Work out the finished part from the listing and answer in its coordinate system (mm). A direction names the side the tool comes from. Give positions to 0.01 mm unless a question says otherwise; leave off trailing zeros. Loops run counter-clockwise (first coordinate to the right, second up) from the corner with the lowest first, then second, coordinate; pieces in that order, holes last. Notation, with made-up numbers: (-30, 5.25) - (3, 5.25) arc R17 cw to (3, 30.25) - close; hole circle Ø7 at (-37.5, 17.25). An arc over 180 degrees is marked (long way). One line per question, with ' | ' between items.
from build123d import *

# Parameters (mm, degrees)
CROQUIS1_R              = 10
SALIENTE_EXTRUIR1_DEPTH = 75
CROQUIS2_R              = 11
SALIENTE_EXTRUIR2_DEPTH = 2
CROQUIS3_W              = 15
CROQUIS3_H              = 10
SALIENTE_EXTRUIR3_DEPTH = 5


with BuildPart() as part:
    # Croquis1 → Saliente-Extruir1 (new body)
    with BuildSketch(Plane.XY):
        Circle(CROQUIS1_R)
    extrude(amount=SALIENTE_EXTRUIR1_DEPTH)

    # Croquis2 → Saliente-Extruir2 (add)
    with BuildSketch(Plane.XY.offset(75)):
        Circle(CROQUIS2_R)
    extrude(amount=SALIENTE_EXTRUIR2_DEPTH)

    # Croquis3 → Saliente-Extruir3 (add)
    with BuildSketch(Plane(origin=(0, 0, 0), x_dir=(-1, 0, 0), z_dir=(0, 0, -1))):
        Rectangle(CROQUIS3_W, CROQUIS3_H)
    extrude(amount=SALIENTE_EXTRUIR3_DEPTH)


solid = part.part
1. Find section C-C on z = 19. Write down the section's boundary in (x, y), then the cut area to 3 significant figures.
Evaluation:
outline: circle Ø20 at (0, 0) | area: 314 mm2
2. Find section D-D on y = 7.25. Write down the section's boundary in (x, z), then the cut area to 3 significant figures.
Evaluation:
outline: (-8.27, 75) - (-6.89, 75) - (-6.89, 0) - (6.89, 0) - (6.89, 75) - (8.27, 75) - (8.27, 77) - (-8.27, 77) - close | area: 1,070 mm2
3. Flat-ended cylindrical pins translate along their axes: pin 1 (5.5 mm diameter, centred on x = 1, z = -2.5, fed in from +Y); pin 2 (1 mm diameter, centred on x = 3, z = 26.5, fed in from -Y); pin 3 (3 mm diameter, centred on y = 6, z = 46, fed in from +X). Find the tip coordinate at first contact, or state that the pin passes through.
Evaluation:
pin 1: y = 10 | pin 2: y = -9.68 | pin 3: x = 8.93
4. Consider L1, parallel to Z at x = -6.75, y = -7.5; L2, parallel to X at y = 0.5, z = 62; L3, parallel to Z at x = 7.75, y = -3.5. Determine where each line is inside the solid, lowest interval first.
Evaluation:
L1: 75 to 77 | L2: -9.99 to 9.99 | L3: 0 to 77
5. Which of the six approach directions +Z, -Z, +X, -X, +Y, -Y give full straight-line access (tool end or side, diameter ignored) to faces 1 (the flat face through (-7.5, 0, -2)), 2 (the flat face through (7.5, 0, -2)), 3 (the cylindrical face through (-2.17, -9.76, 36.98))?
Evaluation:
face 1: -Z, -X, +Y, -Y | face 2: -Z, +X, +Y, -Y | face 3: -Z
6. Find section A-A on x = 0. Write down the section's boundary in (y, z).
Evaluation:
outline: (-11, 75) - (-10, 75) - (-10, 0) - (-5, 0) - (-5, -5) - (5, -5) - (5, 0) - (10, 0) - (10, 75) - (11, 75) - (11, 77) - (-11, 77) - close
7. Find section B-B on y = 0. Write down the section's boundary in (x, z), then the cut area to 3 significant figures.
Evaluation:
outline: (-11, 75) - (-10, 75) - (-10, 0) - (-7.5, 0) - (-7.5, -5) - (7.5, -5) - (7.5, 0) - (10, 0) - (10, 75) - (11, 75) - (11, 77) - (-11, 77) - close | area: 1,620 mm2
